Here's how the part is built. I have some questions about the finished solid (model axes, mm). A direction names the side the tool comes from. Coordinates: 2 decimals unless noted, no trailing zeros. Write each loop counter-clockwise with the first axis right and the second up, starting at its lowest first coordinate (ties: lowest second). Pieces come first, ordered by that corner, then holes.
from build123d import *

# Parameters (mm, degrees)
SKETCH1_W                = 17.5
SKETCH1_H                = 28
BOSS_EXTRUDE1_DEPTH      = 1.6
BOSS_EXTRUDE2_DEPTH      = 1
BOSS_EXTRUDE2_DEPTH_BACK = 6.4
CUT_EXTRUDE1_DEPTH       = 6
SKETCH4_W                = 6.110016504
SKETCH4_H                = 0.488801321
BOSS_EXTRUDE3_DEPTH      = 5


with BuildPart() as part:
    # Sketch1 → Boss-Extrude1 (new body)
    with BuildSketch(Plane(origin=(0, 0, 0), x_dir=(1, 0, 0), z_dir=(0, 1, 0))):
        with Locations((8.75, 14)):
            Rectangle(SKETCH1_W, SKETCH1_H)
    extrude(amount=BOSS_EXTRUDE1_DEPTH)

    # Sketch2 → Boss-Extrude2 (add, two sides: drawn at the far end of the back side and taken through both)
    with BuildSketch(Plane.XY.offset(-BOSS_EXTRUDE2_DEPTH_BACK)):
        with BuildLine():
            Line((5.95, 5), (11.55, 5))
            ThreePointArc((11.55, 5), (13.25, 3.3), (11.55, 1.6))
            Line((11.55, 1.6), (5.95, 1.6))
            ThreePointArc((5.95, 1.6), (4.25, 3.3), (5.95, 5))
        make_face()
    extrude(amount=BOSS_EXTRUDE2_DEPTH + BOSS_EXTRUDE2_DEPTH_BACK)

    # Sketch3 → Cut-Extrude1 (cut)
    with BuildSketch(Plane.XY.offset(1)):
        with BuildLine():
            Line((11.55, 2.3), (5.95, 2.3))
            ThreePointArc((5.95, 2.3), (4.95, 3.3), (5.95, 4.3))
            Line((5.95, 4.3), (11.55, 4.3))
            ThreePointArc((11.55, 4.3), (12.55, 3.3), (11.55, 2.3))
        make_face()
    extrude(amount=-CUT_EXTRUDE1_DEPTH, mode=Mode.SUBTRACT)

    # Sketch4 → Boss-Extrude3 (add)
    with BuildSketch(Plane.XY.offset(-5)):
        with Locations((8.750272331, 3.285790187)):
            Rectangle(SKETCH4_W, SKETCH4_H)
    extrude(amount=BOSS_EXTRUDE3_DEPTH)


solid = part.part
1. If I drill on line 1 (Y direction, x = 11.25, z = -1.75); line 2 (Y direction, x = 11.25, z = -19); line 3 (Z direction, x = 13, y = 0.4), over which ranges is the centre line in solid material (lowest first)?
2. I want a section at A-A (z = -1). List the corners of the cut face in (x, y) for me, then the cut area to 3 significant figures.
3. I want a section at B-B (y = 1.3). List the corners of the cut face in (x, z) for me, then the cut area to 3 significant figures.
4. On a 3-axis mill with a long thin cutter (end or side, diameter ignored), from which of +Z, -Z, +X, -X, +Y, -Y can I reach the whole of each face in a straight line? I mean faces 5 (the face through (9, 3, -6.4)), 6 (the face through (9, 4.3, -2)), 7 (the face through (17.5, 1, -14)). Say none if no direction works.
5. For pin 1 Ø0.6 at (x, y) = (7, 3.5) entering from +Z; pin 2 Ø1.5 at (x, z) = (8.5, -3.5) entering from -Y; pin 3 Ø1 at (x, y) = (2, 4.5) entering from -Z; pin 4 Ø9 at (x, z) = (12, -18.5) entering from +Y, each with a flat end and sliding along its axis, tell me the tip position at first contact or that it passes through.
6. Thinking about a two-plate mould opening in X: for faces 1 (the face through (0, 1, -14)), 2 (the face through (9, 1, 0)), 3 (the face through (12.55, 3.32, -1.96)), 4 (the face through (4.95, 3.28, -1.96)), which applies, pulls with the +X half, pulls with the -X half, needs draft (parallel to the pull), parting line crosses it, or undercut?
7. I want a section at C-C (z = -24.75). List the corners of the cut face in (x, y) for me, then the cut area to 3 significant figures.
Response values:
1. line 1: y = 0 to 2.3, 3.04 to 3.53, 4.3 to 5
1. line 2: y = 0 to 1.6
1. line 3: z = -28 to 0
2. outline: (0, 0) - (17.5, 0) - (17.5, 1.6) - (11.55, 1.6) arc R1.7 ccw to (11.55, 5) - (5.95, 5) arc R1.7 ccw to (5.95, 1.6) - (0, 1.6) - close; (5.7, 3.04) - (11.81, 3.04) - (11.81, 3.53) - (5.7, 3.53) - close; hole (5.95, 2.3) - (11.55, 2.3) arc R1 ccw to (11.55, 4.3) - (5.95, 4.3) arc R1 ccw to start
2. area: 44.8 mm2
3. outline: (0, -28) - (17.5, -28) - (17.5, 0) - (0, 0) - close
3. area: 490 mm2
4. face 5: -Z, +X, -X, +Y
4. face 6: +Z
4. face 7: +Z, -Z, +X, +Y, -Y
5. pin 1: stops at z = 0
5. pin 2: stops at y = 0
5. pin 3: passes through
5. pin 4: stops at y = 1.6
6. face 1: pulls with the -X half
6. face 2: needs draft
6. face 3: undercut
6. face 4: undercut
7. outline: (0, 0) - (17.5, 0) - (17.5, 1.6) - (0, 1.6) - close
7. area: 28.0 mm2
